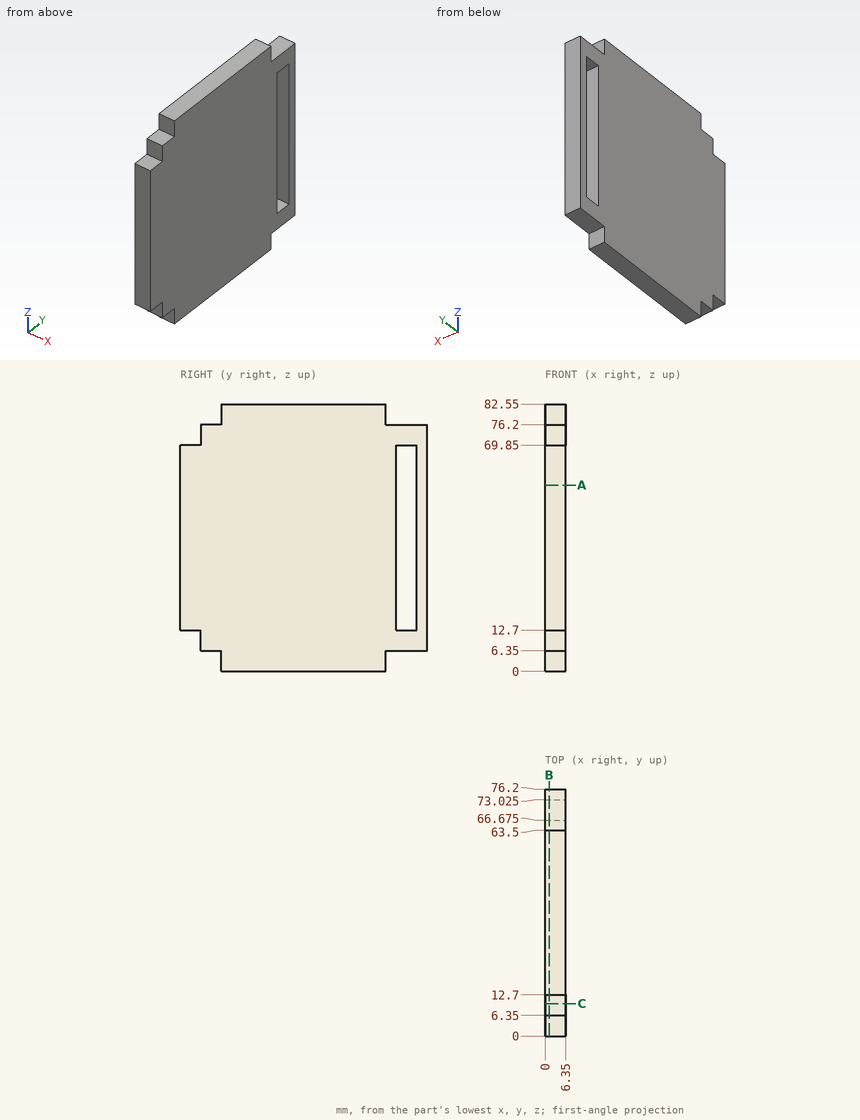
Geometry check sheet. Reference: drawing and pictorial views, mm from the part's lowest x, y, z. Coordinates: 2 decimals unless noted, no trailing zeros. Order: outer loops, then holes, each group sorted by start corner. A loop starts at its lowest first (then second) coordinate and runs counter-clockwise, first axis right, second up. Notation, with made-up numbers: (-25.75, 17.5) - (-9.75, 17.5) arc R21 ccw to (-9.75, 22.5) - close; hole circle Ø5 at (-18, -27.5). An arc over 180 degrees is marked (long way). One line per item, written item: value.
(1) Sectioned sample at C-C (y = 10). Enter the section's corners in (x, z), and give its area (3 significant figures).
Data:
outline: (0, 6.35) - (6.35, 6.35) - (6.35, 76.2) - (0, 76.2) - close
area: 444 mm^2
(2) Sectioned sample at B-B (x = 1.25). Enter the section's corners in (y, z) (3 decimals), and give its area (3 significant figures).
Data:
outline: (0, 12.7) - (6.35, 12.7) - (6.35, 6.35) - (12.7, 6.35) - (12.7, 0) - (63.5, 0) - (63.5, 6.35) - (76.2, 6.35) - (76.2, 76.2) - (63.5, 76.2) - (63.5, 82.55) - (12.7, 82.55) - (12.7, 76.2) - (6.35, 76.2) - (6.35, 69.85) - (0, 69.85) - close; hole (66.675, 12.7) - (73.025, 12.7) - (73.025, 69.85) - (66.675, 69.85) - close
area: 5,520 mm^2
(3) Sectioned sample at A-A (z = 57.5). Enter the section's corners in (x, y) (3 decimals).
Data:
outline: (0, 0) - (6.35, 0) - (6.35, 66.675) - (0, 66.675) - close; (0, 73.025) - (6.35, 73.025) - (6.35, 76.2) - (0, 76.2) - close
(4) Depth check by flat-ended pin: pin 1 Ø5 at (y, z) = (52, 62) entering from -X; pin 2 Ø3 at (x, y) = (4, 9.5) entering from -Z; pin 3 Ø3 at (x, z) = (1.5, 4.5) entering from -Y. Enter the tip coordinate at first touch or a pass-through.
Data:
pin 1: stops at x = 0
pin 2: stops at z = 6.35
pin 3: stops at y = 12.7
(5) Thickness scan on probe 1 along Y at (x, z) = (3, 66) (3 decimals); probe 2 along Z at (x, y) = (2.5, 72.5); probe 3 along Y at (x, z) = (4.75, 10). Record the ranges inside material, lowest first. Write a range as from..to.
Data:
probe 1: y = 0..66.675, 73.025..76.2
probe 2: z = 6.35..12.7, 69.85..76.2
probe 3: y = 6.35..76.2
